Check sheet for the modelled part. Datum: model origin and axes. Units: mm. Face numbers are marked on the shaded views. A direction names the side the tool comes from. Round coordinates to 2 decimals unless told otherwise and drop trailing zeros. Write each loop counter-clockwise with the first axis right and the second up, starting at its lowest first coordinate (ties: lowest second). Pieces come first, ordered by that corner, then holes. Notation, with made-up numbers: M 54,-33.75 L 89,-33.75 A22 ccw 89,-23.75 Z; hole C 77.25,3 d2. An arc over 180 degrees is marked long. One line per item, written item: value.
from build123d import *

# Parameters (mm, degrees)
ESQUISSE1_R        = 10
BOSS_EXTRU_1_DEPTH = 15
ESQUISSE2_R        = 3.5
BOSS_EXTRU_2_DEPTH = 16


with BuildPart() as part:
    # Esquisse1 → Boss.-Extru.1 (new body)
    with BuildSketch(Plane.XY):
        Circle(ESQUISSE1_R)
    extrude(amount=BOSS_EXTRU_1_DEPTH)

    # Esquisse2 → Boss.-Extru.2 (add)
    with BuildSketch(Plane.XY.offset(15)):
        Circle(ESQUISSE2_R)
    extrude(amount=BOSS_EXTRU_2_DEPTH)

    # Esquisse3 → Révolution1 (revolve)
    with BuildSketch(Plane(origin=(0, 0, 0), x_dir=(1, 0, 0), z_dir=(0, 1, 0))):
        with BuildLine():
            Line((0, 3), (0, -9))
            ThreePointArc((0, -9), (6, -3), (0, 3))
        make_face()
    revolve(axis=Axis((0, 0, 34.789870501), (0, 0, -1)))


solid = part.part
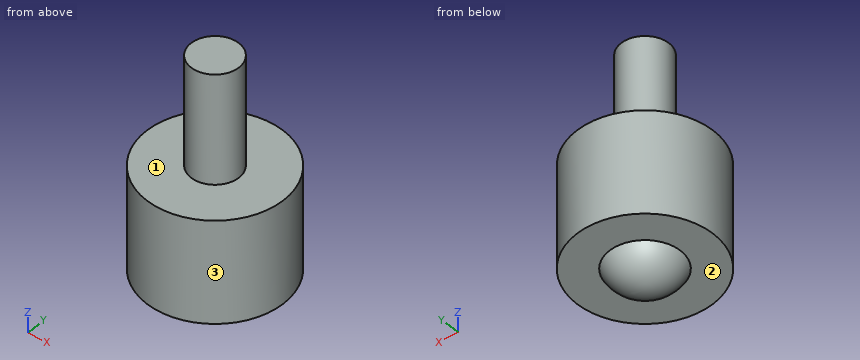
Q1. Access from +Z, -Z, +X, -X, +Y, -Y to the whole of each face (thin tool, end or side, straight path). Record for the marked faces 1, 2 and 3.
Completed:
face 1: +Z
face 2: -Z
face 3: +Z, -Z
Q2. Depth check by flat-ended pin: P1, Ø8, axis at x = -1, y = 8, coming from the +Z side; P2, Ø6, axis at x = -4.5, z = 3, coming from the -Y side; P3, Ø3, axis at x = -4, z = 11, coming from the -Y side. Enter the tip coordinate at first touch or a pass-through.
Completed:
P1: z = 15
P2: y = -9.89
P3: y = -9.68
Q3. Sectioned sample at B-B on x = -1.75. Enter the section's corners in (y, z).
Completed:
outline: M -9.85,0 L -4.89,0 A5.74 ccw 4.89,0 L 9.85,0 L 9.85,15 L 3.03,15 L 3.03,31 L -3.03,31 L -3.03,15 L -9.85,15 Z
Q4. Sectioned sample at C-C on z = 8. Enter the section's corners in (x, y), and give its area (3 significant figures).
Completed:
outline: C 0,0 d20
area: 314 mm^2
Q5. Sectioned sample at D-D on x = -4.25. Enter the section's corners in (y, z), and give its area (3 significant figures).
Completed:
outline: M -9.05,0 L -2.99,0 A4.24 ccw 2.99,0 L 9.05,0 L 9.05,15 L -9.05,15 Z
area: 277 mm^2
Q6. Sectioned sample at A-A on y = 0. Enter the section's corners in (x, z), and give its area (3 significant figures).
Completed:
outline: M -10,0 L -5.2,0 A6 ccw 5.2,0 L 10,0 L 10,15 L 3.5,15 L 3.5,31 L -3.5,31 L -3.5,15 L -10,15 Z
area: 434 mm^2
Q7. Scan lines: line 1 (Z direction, x = -5.5, y = -4.25); line 2 (X direction, y = -0.25, z = 5.5); line 3 (Y direction, x = -7.75, z = 10). Record each from-to range of solid material in increasing order. Write a range as [from, to].
Completed:
line 1: [0, 15]
line 2: [-10, 10]
line 3: [-6.32, 6.32]
